```python
from build123d import *

# Parameters (mm, degrees)
SKETCH1_R                                         = 85.725
BOSS_EXTRUDE1_DEPTH                               = 6.35
SKETCH2_R                                         = 6.35
BOSS_EXTRUDE2_DEPTH                               = 26.67
SKETCH6_R                                         = 22.86
CUT_EXTRUDE1_DEPTH                                = 6.35
CUT_EXTRUDE3_REACH                                = 126.132
SKETCH10_R                                        = 19.05
SKETCH11_R                                        = 9.525
BOSS_EXTRUDE3_DEPTH                               = 9.525
SKETCH12_W                                        = 1.905
SKETCH12_H                                        = 1.27
CIRPATTERN6_COUNT                                 = 3
CIRPATTERN7_COUNT                                 = 3
CHAMFER2_SIZE                                     = 1.27
SKETCH13_W                                        = 38.1
SKETCH13_H                                        = 54.266652261
BOSS_EXTRUDE5_DEPTH                               = 6.35
CIRPATTERN8_COUNT                                 = 3
FILLET1_RADIUS                                    = 19.05
FILLET1_LENGTH                                    = 6.35
BOSS_EXTRUDE9_DEPTH                               = 6.35
CSK_FOR_8_FLAT_HEAD_MACHINE_SCREW_100_D           = 4.4958
CSK_FOR_8_FLAT_HEAD_MACHINE_SCREW_100_CSINK_D     = 8.4328
CSK_FOR_8_FLAT_HEAD_MACHINE_SCREW_100_CSINK_ANGLE = 100
F_1_2_0_5_DIAMETER_HOLE2_D                        = 12.7
MIRROR3_COPY_1_DEPTH                              = 6.35
FILLET1_OF_MIRROR3_2_RADIUS                       = 19.05
FILLET1_OF_MIRROR3_2_LENGTH                       = 6.35
CHAMFER3_SIZE                                     = 1.27


with BuildPart() as part:
    # Sketch1 → Boss-Extrude1 (new body)
    with BuildSketch(Plane.XY):
        Circle(SKETCH1_R)
    extrude(amount=BOSS_EXTRUDE1_DEPTH)

    # Sketch2 → Boss-Extrude2 (add)
    with BuildSketch(Plane.XY):
        with Locations((41.794385987, -24.13)):
            Circle(SKETCH2_R)
        with Locations((0, 48.26)):
            Circle(SKETCH2_R)
        with Locations((-41.794385987, -24.13)):
            Circle(SKETCH2_R)
    extrude(amount=BOSS_EXTRUDE2_DEPTH)

    # Sketch6 → Cut-Extrude1 (cut)
    with BuildSketch(Plane.XY):
        Circle(SKETCH6_R)
    extrude(amount=CUT_EXTRUDE1_DEPTH, mode=Mode.SUBTRACT)

    # Sketch10 → Cut-Extrude3 (cut, up to next)
    with BuildSketch(Plane.XY, mode=Mode.PRIVATE) as cut_extrude3_sk1:
        with Locations((43.994090512, 25.4)):
            Circle(SKETCH10_R)
    cut_extrude3_tool1 = extrude(cut_extrude3_sk1.sketch, amount=CUT_EXTRUDE3_REACH, mode=Mode.PRIVATE) & part.part
    cut_extrude3 = cut_extrude3_tool1.solids().sort_by_distance((43.994091, 25.4, 0))[0]
    add(cut_extrude3, mode=Mode.SUBTRACT)

    # Sketch11 → Boss-Extrude3 (add)
    with BuildSketch(Plane.XY):
        with Locations(Location((0, 48.26, 0), (0, 0, 180))):
            Circle(SKETCH11_R)
    boss_extrude3 = extrude(amount=BOSS_EXTRUDE3_DEPTH)

    # Sketch12 → Cut-Revolve1 (revolve, cut)
    with BuildSketch(Plane(origin=(0, 0, 0), x_dir=(0, 0, -1), z_dir=(1, 0, 0)), mode=Mode.PRIVATE) as cut_revolve1_sk:
        with Locations((-24.4475, 54.61)):
            Rectangle(SKETCH12_W, SKETCH12_H)
    cut_revolve1 = revolve(cut_revolve1_sk.sketch.rotate(Axis((0, 48.26, 26.67), (0, 0, 1)), 90), axis=Axis((0, 48.26, 26.67), (0, 0, 1)), mode=Mode.SUBTRACT)

    # CirPattern6: Boss-Extrude3 ×3 about axis
    cirpattern6_axis = Axis((0, 0, 0), (0, 0, 1))
    for i in range(1, CIRPATTERN6_COUNT):
        add(boss_extrude3.rotate(cirpattern6_axis, i * 360 / CIRPATTERN6_COUNT))

    # CirPattern7: Cut-Revolve1 ×3 about axis
    cirpattern7_axis = Axis((0, 0, 0), (0, 0, 1))
    for i in range(1, CIRPATTERN7_COUNT):
        add(cut_revolve1.rotate(cirpattern7_axis, i * 360 / CIRPATTERN7_COUNT), mode=Mode.SUBTRACT)

    # Chamfer2
    chamfer2_edges = [part.edges().sort_by_distance(p)[0] for p in [
        (-85.725, 0, 0),
        (9.525, 48.26, 6.35),
        (-46.556885987, -15.881108029, 6.35),
        (-85.725, 0, 6.35),
        (37.031885987, -32.378891971, 6.35),
    ]]
    chamfer(chamfer2_edges, length=CHAMFER2_SIZE)

    # Sketch13 → Boss-Extrude5 (add)
    with BuildSketch(Plane.XY):
        with Locations((0, 109.411783366)):
            Rectangle(SKETCH13_W, SKETCH13_H)
    boss_extrude5 = extrude(amount=BOSS_EXTRUDE5_DEPTH)

    # CirPattern8: Cut-Extrude3 ×3 about axis
    cirpattern8_axis = Axis((0, 0, 0), (0, 0, 1))
    for i in range(1, CIRPATTERN8_COUNT):
        add(cut_extrude3.rotate(cirpattern8_axis, i * 360 / CIRPATTERN8_COUNT), mode=Mode.SUBTRACT)

    # Fillet1: full round fillet: the end face becomes a half cylinder, R = half its width
    fillet1_face = Plane((0, 136.545109496, 3.175), x_dir=(0, 0, -1), z_dir=(0, 1, 0))  # on the end face: x along it, z out of the body
    fillet1_slab = fillet1_face.offset(-FILLET1_RADIUS / 2) * Box(FILLET1_LENGTH, 2 * FILLET1_RADIUS, FILLET1_RADIUS, mode=Mode.PRIVATE)  # the body's end, R deep
    fillet1_round = Plane((0, 117.495109496, 3.175), x_dir=(0, 1, 0), z_dir=(0, 0, -1)) * Cylinder(FILLET1_RADIUS, FILLET1_LENGTH, mode=Mode.PRIVATE)  # its axis R under the face
    add(fillet1_slab - fillet1_round, mode=Mode.SUBTRACT)

    # Sketch25 → Boss-Extrude9 (add)
    with BuildSketch(Plane.XY):
        with BuildLine():
            Line((-19.05, 96.237596733), (-19.05, 82.278457235))
            ThreePointArc((-19.05, 82.278457235), (-25.139009769, 80.626777269), (-31.087730061, 78.525155617))
            ThreePointArc((-31.087730061, 78.525155617), (-22.344267038, 85.52968476), (-19.05, 96.237596733))
        make_face()
    boss_extrude9 = extrude(amount=BOSS_EXTRUDE9_DEPTH)

    # Mirror1: Boss-Extrude9 across plane
    add(boss_extrude9.mirror(Plane(origin=(0, 0, 0), x_dir=(0, 0, 1), z_dir=(1, 0, 0))))

    # CSK for #8 Flat Head Machine Screw (100)2 (through all)
    with Locations(Plane.XY.offset(6.35)):
        with Locations((-12.7, 97.602206046), (12.7, 97.602206046)):
            csk_for_8_flat_head_machine_screw_100 = CounterSinkHole(CSK_FOR_8_FLAT_HEAD_MACHINE_SCREW_100_D / 2, CSK_FOR_8_FLAT_HEAD_MACHINE_SCREW_100_CSINK_D / 2, counter_sink_angle=CSK_FOR_8_FLAT_HEAD_MACHINE_SCREW_100_CSINK_ANGLE)

    # 1/2 (0.5) Diameter Hole2 (through all)
    with Locations(Plane.XY.offset(6.35)):
        with Locations((0, 117.495109496)):
            f_1_2_0_5_diameter_hole2 = Hole(F_1_2_0_5_DIAMETER_HOLE2_D / 2)

    # Mirror3: Boss-Extrude5, Boss-Extrude9, CSK for #8 Flat Head Machine Screw (100)2, 1/2 (0.5) Diameter Hole2 across plane
    add(boss_extrude5.mirror(Plane.ZX))
    add(boss_extrude9.mirror(Plane.ZX))
    add(csk_for_8_flat_head_machine_screw_100.mirror(Plane.ZX), mode=Mode.SUBTRACT)
    add(f_1_2_0_5_diameter_hole2.mirror(Plane.ZX), mode=Mode.SUBTRACT)

    # Mirror3 copy 1 sketch → Mirror3 copy 1 (add)
    with BuildSketch(Plane(origin=(0, 0, 0), x_dir=(-1, 0, 0), z_dir=(0, 0, 1))):
        with BuildLine():
            Line((-19.05, 96.237596733), (-19.05, 82.278457235))
            ThreePointArc((-19.05, 82.278457235), (-25.139009769, 80.626777269), (-31.087730061, 78.525155617))
            ThreePointArc((-31.087730061, 78.525155617), (-22.344267038, 85.52968476), (-19.05, 96.237596733))
        make_face()
    extrude(amount=MIRROR3_COPY_1_DEPTH)

    # Fillet1 of Mirror3 2: full round fillet: the end face becomes a half cylinder, R = half its width
    fillet1_of_mirror3_2_face = Plane((0, -136.545109496, 3.175), x_dir=(0, 0, -1), z_dir=(0, -1, 0))  # on the end face: x along it, z out of the body
    fillet1_of_mirror3_2_slab = fillet1_of_mirror3_2_face.offset(-FILLET1_OF_MIRROR3_2_RADIUS / 2) * Box(FILLET1_OF_MIRROR3_2_LENGTH, 2 * FILLET1_OF_MIRROR3_2_RADIUS, FILLET1_OF_MIRROR3_2_RADIUS, mode=Mode.PRIVATE)  # the body's end, R deep
    fillet1_of_mirror3_2_round = Plane((0, -117.495109496, 3.175), x_dir=(0, -1, 0), z_dir=(0, 0, -1)) * Cylinder(FILLET1_OF_MIRROR3_2_RADIUS, FILLET1_OF_MIRROR3_2_LENGTH, mode=Mode.PRIVATE)  # its axis R under the face
    add(fillet1_of_mirror3_2_slab - fillet1_of_mirror3_2_round, mode=Mode.SUBTRACT)

    # Chamfer3
    chamfer3_edges = [part.edges().sort_by_distance(p)[0] for p in [
        (-19.05, 106.866353115, 6.35),
        (-19.05, 106.866353115, 0),
        (0, 136.545109496, 6.35),
        (0, 136.545109496, 0),
        (-22.344267038, 85.52968476, 0),
        (-22.344267038, 85.52968476, 6.35),
        (19.05, 106.866353115, 0),
        (19.05, 106.866353115, 6.35),
        (22.344267038, 85.52968476, 6.35),
        (22.344267038, 85.52968476, 0),
        (-19.05, -106.866353115, 6.35),
        (-19.05, -106.866353115, 0),
        (0, -136.545109496, 0),
        (0, -136.545109496, 6.35),
        (-22.344267038, -85.52968476, 6.35),
        (-22.344267038, -85.52968476, 0),
        (19.05, -106.866353115, 6.35),
        (19.05, -106.866353115, 0),
        (22.344267038, -85.52968476, 0),
        (22.344267038, -85.52968476, 6.35),
    ]]
    chamfer(chamfer3_edges, length=CHAMFER3_SIZE)


solid = part.part
```
Geometry check sheet. Reference: the model listing, model coordinates, mm. A direction names the side the tool comes from. Coordinates: 2 decimals unless noted, no trailing zeros. Loops run counter-clockwise (first coordinate to the right, second up) from the corner with the lowest first, then second, coordinate; pieces in that order, holes last.
Item 1: Release check for a two-part mould opening along Z. For faces 4 (the face through (20.84, 88.18, 3.15)), 5 (the face through (42, -18, 23.495)), 6 (the face through (0, 48, 26.67)) record: released by +Z, released by -Z, zero draft, split by the parting line, or undercut.
Item 2: Sectioned sample at A-A, the plane y = 0. Record the boundary of the cut face in (x, z) (3 decimals), then the cut area to 3 significant figures.
Item 3: Thickness scan on line 1 (Y direction, x = 0, z = 2.25); line 2 (Y direction, x = 13, z = 4.25); line 3 (X direction, y = 25.4, z = 3.75). Record the ranges inside material, lowest first.
Item 4: Access from +Z, -Z, +X, -X, +Y, -Y to the whole of each face (thin tool, end or side, straight path). Record for faces 1 (the face through (-20.581, -87.92, 0.926)), 2 (the face through (42, -18, 25.4)), 3 (the face through (-35.74, -22.22, 16.41)).
Item 5: Go/stop test with flat-tipped pins: pin 1 Ø4 at (x, z) = (-49, 15.5) entering from +Y; pin 2 Ø1.5 at (x, z) = (62, 3) entering from -Y; pin 3 Ø4 at (y, z) = (-107, 4) entering from +X. Record where each tip stops, or that it passes through.
Item 6: Sectioned sample at B-B, the plane z = 12.25. Record the boundary of the cut face in (x, y).
Item 7: Sectioned sample at C-C, the plane x = 0. Count the separate pieces of the cut face and the enclosed holes in it, then the cut area to 3 significant figures.
Check result:
1. face 4: zero draft
1. face 5: undercut
1. face 6: released by +Z
2. outline: (-85.725, 1.27) - (-84.455, 0) - (-22.86, 0) - (-22.86, 6.35) - (-84.455, 6.35) - (-85.725, 5.08) - close; (22.86, 0) - (84.455, 0) - (85.725, 1.27) - (85.725, 5.08) - (84.455, 6.35) - (22.86, 6.35) - close
2. area: 795 mm2
3. line 1: y = -136.55 to -123.85, -111.15 to -69.85, -31.75 to -22.86, 22.86 to 111.15, 123.85 to 136.55
3. line 2: y = -131.42 to -99.83, -95.37 to -64.72, -36.88 to -18.8, 18.8 to 95.37, 99.83 to 131.42
3. line 3: x = -81.88 to -63.04, -24.94 to 24.94, 63.04 to 81.88
4. face 1: -Z, -X, -Y
4. face 2: none
4. face 3: +Z
5. pin 1: stops at y = -20.49
5. pin 2: stops at y = -59.98
5. pin 3: stops at x = 19.05
6. outline: circle Ø12.7 at (-41.79, -24.13); circle Ø12.7 at (0, 48.26); circle Ø12.7 at (41.79, -24.13)
7. separate pieces: 5
7. enclosed holes: 0
7. area: 1,310 mm2
